from build123d import *

# Parameters (mm, degrees)
SKETCH1_R           = 1.5
BOSS_EXTRUDE1_DEPTH = 43.75
SKETCH2_OUTSIDE_W   = 13.792
SKETCH2_OUTSIDE_H   = 13.792
SKETCH2_OUTSIDE_R   = 1
CUT_EXTRUDE1_DEPTH  = 3.5
SKETCH3_OUTSIDE_W   = 13.792
SKETCH3_OUTSIDE_H   = 13.792
SKETCH3_OUTSIDE_R   = 0.7
CUT_EXTRUDE2_DEPTH  = 2
SKETCH4_OUTSIDE_W   = 13.792
SKETCH4_OUTSIDE_H   = 13.792
SKETCH4_OUTSIDE_R   = 1
CUT_EXTRUDE5_DEPTH  = 3.5
SKETCH5_OUTSIDE_W   = 13.792
SKETCH5_OUTSIDE_H   = 13.792
SKETCH5_OUTSIDE_R   = 0.7
CUT_EXTRUDE6_DEPTH  = 2
LPATTERN1_COUNT     = 4
LPATTERN1_PITCH     = 1
CHAMFER3_SIZE       = 0.2
CHAMFER4_SIZE       = 0.05


with BuildPart() as part:
    # Sketch1 → Boss-Extrude1 (new body)
    with BuildSketch(Plane(origin=(0, 0, 0), x_dir=(1, 0, 0), z_dir=(0, 1, 0))):
        Circle(SKETCH1_R)
    extrude(amount=BOSS_EXTRUDE1_DEPTH)

    # Sketch2 outside → Cut-Extrude1 (cut)
    with BuildSketch(Plane(origin=(0, 43.75, 0), x_dir=(1, 0, 0), z_dir=(0, 1, 0))):
        Rectangle(SKETCH2_OUTSIDE_W, SKETCH2_OUTSIDE_H)
        Circle(SKETCH2_OUTSIDE_R, mode=Mode.SUBTRACT)
    extrude(amount=-CUT_EXTRUDE1_DEPTH, mode=Mode.SUBTRACT)

    # Sketch3 outside → Cut-Extrude2 (cut)
    with BuildSketch(Plane(origin=(0, 43.75, 0), x_dir=(1, 0, 0), z_dir=(0, 1, 0))):
        Rectangle(SKETCH3_OUTSIDE_W, SKETCH3_OUTSIDE_H)
        Circle(SKETCH3_OUTSIDE_R, mode=Mode.SUBTRACT)
    extrude(amount=-CUT_EXTRUDE2_DEPTH, mode=Mode.SUBTRACT)

    # Sketch4 outside → Cut-Extrude5 (cut)
    with BuildSketch(Plane.XZ):
        Rectangle(SKETCH4_OUTSIDE_W, SKETCH4_OUTSIDE_H)
        Circle(SKETCH4_OUTSIDE_R, mode=Mode.SUBTRACT)
    extrude(amount=-CUT_EXTRUDE5_DEPTH, mode=Mode.SUBTRACT)

    # Sketch5 outside → Cut-Extrude6 (cut)
    with BuildSketch(Plane.XZ):
        Rectangle(SKETCH5_OUTSIDE_W, SKETCH5_OUTSIDE_H)
        Circle(SKETCH5_OUTSIDE_R, mode=Mode.SUBTRACT)
    extrude(amount=-CUT_EXTRUDE6_DEPTH, mode=Mode.SUBTRACT)

    # Sketch6 → Cut-Revolve1 (revolve, cut)
    with BuildSketch(Plane.XY):
        Polygon((-1.5, 23.475), (-1.4, 23.375), (-1.5, 23.275), align=None)
    cut_revolve1 = revolve(axis=Axis((0, 43.75, 0), (0, -1, 0)), mode=Mode.SUBTRACT)

    # LPattern1: Cut-Revolve1 ×4
    with Locations(*[(0, -i * LPATTERN1_PITCH, 0) for i in range(1, LPATTERN1_COUNT)]):
        add(cut_revolve1, mode=Mode.SUBTRACT)

    # Chamfer3
    chamfer3_edges = [part.edges().sort_by_distance(p)[0] for p in [
        (-0.7, 43.75, 0),
        (-0.7, 0, 0),
    ]]
    chamfer(chamfer3_edges, length=CHAMFER3_SIZE)

    # Chamfer4
    chamfer4_edges = [part.edges().sort_by_distance(p)[0] for p in [
        (-1.5, 3.5, 0),
        (-1.5, 40.25, 0),
    ]]
    chamfer(chamfer4_edges, length=CHAMFER4_SIZE)


solid = part.part
Check sheet for the modelled part. Datum: model origin and axes. Units: mm. A direction names the side the tool comes from. Give positions to 0.01 mm unless a question says otherwise; leave off trailing zeros. Loops run counter-clockwise (first coordinate to the right, second up) from the corner with the lowest first, then second, coordinate; pieces in that order, holes last. Notation, with made-up numbers: M -26.75,30.5 L -3.75,30.5 A27 ccw -3.75,52.5 Z; hole C -11.5,-23.75 d6. An arc over 180 degrees is marked long. Answer as a JSON object with one key per item and string values. Group by question number.
Q1. Material ranges on line 1 along Y through (x, z) = (0.85, 0.8); line 2 along Y through (x, z) = (-0.75, 0.2); line 3 along X through (y, z) = (33, 0.4), recorded low to high. Write a range as [from, to].
Q2. Cross-section at A-A on y = 25. Record the cut outline in (x, z).
Q3. Go/stop test with a flat-tipped pin: P1, Ø1.5, axis at x = -1, y = 9, coming from the +Z side. Record where the tip stops, or that it passes through.
Q4. Access from +Z, -Z, +X, -X, +Y, -Y to the whole of each face (thin tool, end or side, straight path). Record for faces 1 (the flat face through (0, 0, 0)), 2 (the cylindrical face through (0, 41, 1)), 3 (the cylindrical face through (0, 3, -1)).
Evaluation:
{
 "1": {"line 1": "y = [3.5, 40.25]", "line 2": "y = [2, 41.75]", "line 3": "x = [-1.45, 1.45]"},
 "2": {"outline": "C 0,0 d3"},
 "3": {"P1": "stops at z = 1.48"},
 "4": {"face 1": "+Z, -Z, +X, -X, -Y", "face 2": "+Y", "face 3": "-Y"}
}
